Read the model definition and answer for the solid it produces. Units are mm, in the model's axes. A direction names the side the tool comes from. Round coordinates to 2 decimals unless told otherwise and drop trailing zeros. Order: outer loops, then holes, each group sorted by start corner. A loop starts at its lowest first (then second) coordinate and runs counter-clockwise, first axis right, second up. Notation, with made-up numbers: (11, 29) - (22, 29) arc R13 cw to (22, 42) - close; hole circle Ø2 at (20, -16). An arc over 180 degrees is marked (long way). Answer as a JSON object with one key per item and string values. Group by question number.
Q1. A cutting plane is placed at C-C on y = -18. Determine the outline of the cut face in (x, z).
Q2. A cutting plane is placed at B-B on x = 11.5. Determine the outline of the cut face in (y, z).
Q3. A tool of negligible diameter and unlimited length cuts with its end or side. For faces 5 (the cylindrical face through (24.33, -18.25, 1.48)), 6 (the cylindrical face through (-10.67, 39.5, 1.48)), 7 (the flat face through (1.9, -25, 2)), from which of +Z, -Z, +X, -X, +Y, -Y can it reach the whole face along a straight path? Write none if from no direction.
Q4. A cutting plane is placed at A-A on z = 2.05. Determine the outline of the cut face in (x, y).
Q5. The mould has two halves that part along Y. Classify faces 1 (the flat face through (36.9, 34, 2)), 2 (the flat face through (12, 24, 0)), 3 (the flat face through (12, 41, 2)), 4 (the cylindrical face through (40.389, 81.886, 1.479)): pulls with the +Y half, pulls with the -Y half, needs draft (parallel to the pull), parting line crosses it, or undercut.
Q6. Given pin 1 Ø1 at (x, z) = (-3.5, 2) entering from -Y, flat-ended and moving along its own axis, determine where the tip first touches the part or whether it passes through.
Q7. Consider line 1 (Y direction, x = 28.9, z = 1.5); line 2 (Y direction, x = 12.4, z = 0.6); line 3 (X direction, y = 75.5, z = 1.3). Determine where each line is inside the solid, lowest interval first.
```python
from build123d import *

# Parameters (mm, degrees)
SKETCH2_W           = 200
SKETCH2_H           = 200
BOSS_EXTRUDE1_DEPTH = 3
SKETCH3_R           = 2.5
CUT_EXTRUDE1_DEPTH  = 10
CUT_EXTRUDE2_REACH  = 143.453
SKETCH4_W           = 200
SKETCH4_H           = 200
SKETCH4_W_2         = 49
SKETCH4_H_2         = 13
FILLET1_R           = 15
FILLET2_R           = 5
CUT_EXTRUDE4_REACH  = 99.207
SKETCH6_R           = 1.6


with BuildPart() as part:
    # Sketch2 → Boss-Extrude1 (new body)
    with BuildSketch(Plane.XY):
        Rectangle(SKETCH2_W, SKETCH2_H)
    extrude(amount=BOSS_EXTRUDE1_DEPTH)

    # Sketch3 → Cut-Extrude1 (cut)
    with BuildSketch(Plane(origin=(0, 0, 0), x_dir=(-1, 0, 0), z_dir=(0, 0, -1))):
        with Locations((-32.4, 11.65)):
            Circle(SKETCH3_R)
        with Locations((7.6, 11.65)):
            Circle(SKETCH3_R)
        with Locations((-12.4, -28.75)):
            Circle(SKETCH3_R)
    extrude(amount=-CUT_EXTRUDE1_DEPTH, mode=Mode.SUBTRACT)

    # Sketch4 → Cut-Extrude2 (cut, up to next)
    with BuildSketch(Plane.XY.offset(3), mode=Mode.PRIVATE) as cut_extrude2_sk1:
        Rectangle(SKETCH4_W, SKETCH4_H)
        with BuildLine():
            Line((-20.1, -16.75), (-20.1, 86.163533864))
            Line((-20.1, 86.163533864), (44.9, 86.163533864))
            Line((44.9, 86.163533864), (44.9, -16.75))
            Line((44.9, -16.75), (22.9, -16.75))
            Line((22.9, -16.75), (22.9, -28.75))
            ThreePointArc((22.9, -28.75), (12.4, -39.25), (1.9, -28.75))
            Line((1.9, -28.75), (1.9, -16.75))
            Line((1.9, -16.75), (-20.1, -16.75))
        make_face(mode=Mode.SUBTRACT)
    cut_extrude2_tool1 = extrude(cut_extrude2_sk1.sketch, amount=-CUT_EXTRUDE2_REACH, mode=Mode.PRIVATE) & part.part
    # Sketch4 → Cut-Extrude2 (cut, up to next)
    with BuildSketch(Plane.XY.offset(3), mode=Mode.PRIVATE) as cut_extrude2_sk2:
        with Locations((12.4, 34.5)):
            Rectangle(SKETCH4_W_2, SKETCH4_H_2)
    cut_extrude2_tool2 = extrude(cut_extrude2_sk2.sketch, amount=-CUT_EXTRUDE2_REACH, mode=Mode.PRIVATE) & part.part
    add(cut_extrude2_tool1.solids().sort_by_distance((0, 97.171573, 3))[0], mode=Mode.SUBTRACT)
    add(cut_extrude2_tool2.solids().sort_by_distance((12.4, 34.5, 3))[0], mode=Mode.SUBTRACT)

    # Fillet1
    fillet1_edges = [part.edges().sort_by_distance(p)[0] for p in [
        (44.9, -16.75, 1.5),
        (44.9, 86.163533864, 1.5),
        (-20.1, 86.163533864, 1.5),
        (-20.1, -16.75, 1.5),
    ]]
    fillet(fillet1_edges, radius=FILLET1_R)

    # Fillet2
    fillet2_edges = [part.edges().sort_by_distance(p)[0] for p in [
        (36.9, 41, 1.5),
        (36.9, 28, 1.5),
        (-12.1, 28, 1.5),
        (-12.1, 41, 1.5),
        (22.9, -16.75, 1.5),
        (1.9, -16.75, 1.5),
    ]]
    fillet(fillet2_edges, radius=FILLET2_R)

    # Sketch6 → Cut-Extrude4 (cut, up to next)
    with BuildSketch(Plane.XY.offset(3), mode=Mode.PRIVATE) as cut_extrude4_sk1:
        with Locations((-4.1, 75.5)):
            Circle(SKETCH6_R)
    cut_extrude4_tool1 = extrude(cut_extrude4_sk1.sketch, amount=-CUT_EXTRUDE4_REACH, mode=Mode.PRIVATE) & part.part
    # Sketch6 → Cut-Extrude4 (cut, up to next)
    with BuildSketch(Plane.XY.offset(3), mode=Mode.PRIVATE) as cut_extrude4_sk2:
        with Locations((28.9, 75.5)):
            Circle(SKETCH6_R)
    cut_extrude4_tool2 = extrude(cut_extrude4_sk2.sketch, amount=-CUT_EXTRUDE4_REACH, mode=Mode.PRIVATE) & part.part
    add(cut_extrude4_tool1.solids().sort_by_distance((-4.1, 75.5, 3))[0], mode=Mode.SUBTRACT)
    add(cut_extrude4_tool2.solids().sort_by_distance((28.9, 75.5, 3))[0], mode=Mode.SUBTRACT)


solid = part.part
```
Result set:
{
 "1": {"outline": "(0.21, 0) - (24.59, 0) - (24.59, 3) - (0.21, 3) - close"},
 "2": {"outline": "(-39.21, 0) - (-31.08, 0) - (-31.08, 3) - (-39.21, 3) - close; (-26.42, 0) - (28, 0) - (28, 3) - (-26.42, 3) - close; (41, 0) - (86.16, 0) - (86.16, 3) - (41, 3) - close"},
 "3": {"face 5": "+Z, -Z, +X, -Y", "face 6": "+Z, -Z", "face 7": "+Z, -Z, -X, -Y"},
 "4": {"outline": "(-20.1, -1.75) arc R15 ccw to (-5.1, -16.75) - (-3.1, -16.75) arc R5 cw to (1.9, -21.75) - (1.9, -28.75) arc R10.5 ccw to (22.9, -28.75) - (22.9, -21.75) arc R5 cw to (27.9, -16.75) - (29.9, -16.75) arc R15 ccw to (44.9, -1.75) - (44.9, 71.16) arc R15 ccw to (29.9, 86.16) - (-5.1, 86.16) arc R15 ccw to (-20.1, 71.16) - close; hole (-12.1, 33) arc R5 ccw to (-7.1, 28) - (31.9, 28) arc R5 ccw to (36.9, 33) - (36.9, 36) arc R5 ccw to (31.9, 41) - (-7.1, 41) arc R5 ccw to (-12.1, 36) - close; hole circle Ø5 at (-7.6, 11.65); hole circle Ø3.2 at (-4.1, 75.5); hole circle Ø5 at (12.4, -28.75); hole circle Ø3.2 at (28.9, 75.5); hole circle Ø5 at (32.4, 11.65)"},
 "5": {"face 1": "undercut", "face 2": "needs draft", "face 3": "undercut", "face 4": "pulls with the +Y half"},
 "6": {"pin 1": "stops at y = -16.75"},
 "7": {"line 1": "y = -16.75 to 28, 41 to 73.9, 77.1 to 86.16", "line 2": "y = -39.25 to -31.25, -26.25 to 28, 41 to 86.16", "line 3": "x = -19.46 to -5.7, -2.5 to 27.3, 30.5 to 44.26"}
}
